The figure shows three views and two pictorial views of one solid part (mm, origin at its lowest corner). Answer the questions. A direction names the side the tool comes from. Coordinates: 2 decimals unless noted, no trailing zeros. Write each loop counter-clockwise with the first axis right and the second up, starting at its lowest first coordinate (ties: lowest second). Pieces come first, ordered by that corner, then holes.
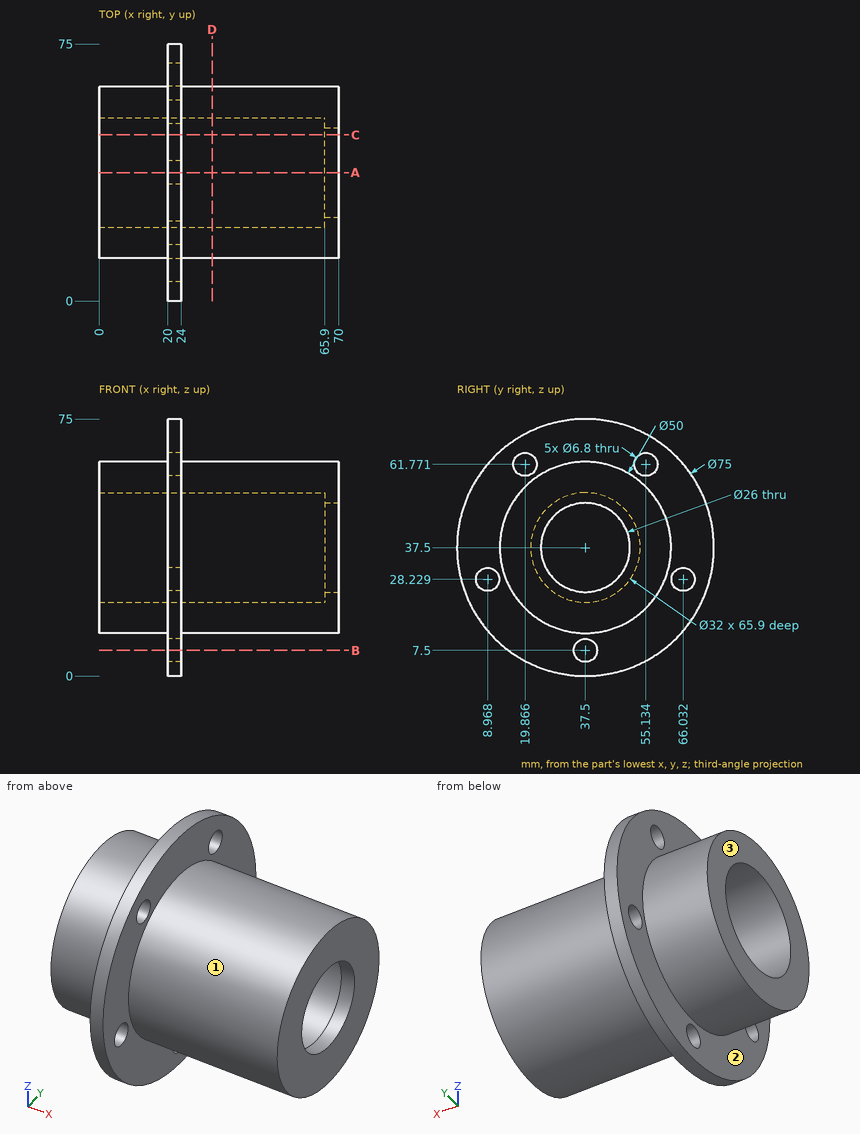
1. Section C-C on y = 48.5 is taken. Give the vertices of the cut face in (x, z).
Results found:
outline: (0, 15.05) - (20, 15.05) - (20, 1.65) - (24, 1.65) - (24, 15.05) - (70, 15.05) - (70, 30.57) - (65.9, 30.57) - (65.9, 25.88) - (0, 25.88) - close; (0, 49.12) - (65.9, 49.12) - (65.9, 44.43) - (70, 44.43) - (70, 59.95) - (24, 59.95) - (24, 73.35) - (20, 73.35) - (20, 59.95) - (0, 59.95) - close
2. Section B-B on z = 7.5 is taken. Give the vertices of the cut face in (x, y).
Results found:
outline: (20, 15) - (24, 15) - (24, 34.1) - (20, 34.1) - close; (20, 40.9) - (24, 40.9) - (24, 60) - (20, 60) - close
3. Find the intervals of material crossed by L1, parallel to Z at x = 21.5, y = 37.5; L2, parallel to Z at x = 25, y = 37.5; L3, parallel to Z at x = 6.5, y = 26 (1 decimal), in increasing order.
Results found:
L1: z = 0 to 4.1, 10.9 to 21.5, 53.5 to 75
L2: z = 12.5 to 21.5, 53.5 to 62.5
L3: z = 15.3 to 26.4, 48.6 to 59.7
4. Flat-ended cylindrical pins translate along their axes: P1, Ø4, axis at x = 27.5, z = 25.5, coming from the +Y side; P2, Ø1.5, axis at y = 45, z = 13.5, coming from the +X side; P3, Ø3, axis at x = 17.5, y = 38, coming from the -Z side; P4, Ø8, axis at x = 29, y = 54.5, coming from the +Z side (1 decimal). Find the tip coordinate at first contact, or state that the pin passes through.
Results found:
P1: stops at y = 60.41
P2: stops at x = 70
P3: stops at z = 12.5
P4: stops at z = 58.9
5. A tool of negligible diameter and unlimited length cuts with its end or side. For the marked faces 1, 2 and 3, from which of +Z, -Z, +X, -X, +Y, -Y can it reach the whole face along a straight path? Write none if from no direction.
Results found:
face 1: +X
face 2: -X
face 3: +Z, -Z, -X, +Y, -Y
6. Section A-A on y = 37.5 is taken. Give the vertices of the cut face in (x, z), then the cut area to 3 significant figures.
Results found:
outline: (0, 12.5) - (20, 12.5) - (20, 10.9) - (24, 10.9) - (24, 12.5) - (70, 12.5) - (70, 24.5) - (65.9, 24.5) - (65.9, 21.5) - (0, 21.5) - close; (0, 53.5) - (65.9, 53.5) - (65.9, 50.5) - (70, 50.5) - (70, 62.5) - (24, 62.5) - (24, 75) - (20, 75) - (20, 62.5) - (0, 62.5) - close; (20, 0) - (24, 0) - (24, 4.1) - (20, 4.1) - close
area: 1,360 mm2
7. Section D-D on x = 33 is taken. Give the vertices of the cut face in (y, z).
Results found:
outline: circle Ø50 at (37.5, 37.5); hole circle Ø32 at (37.5, 37.5)
